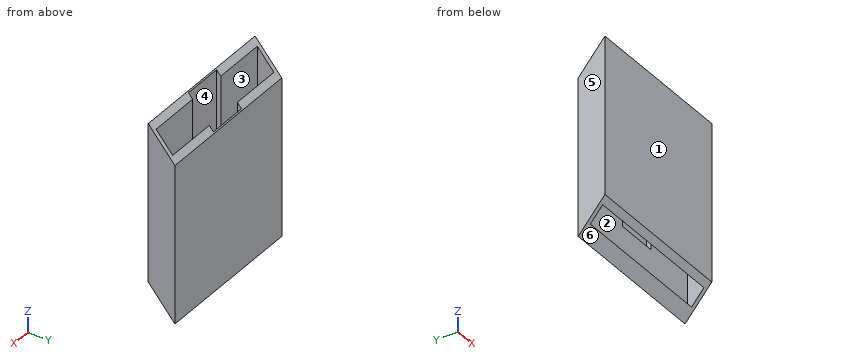
```python
from build123d import *

# Parameters (mm, degrees)
F1_DEPTH = 24.13
F2_W     = 12.7
F2_H     = 1.27
F3_DEPTH = 45.72
F4_DEPTH = 54.61


with BuildPart() as f1:
    # F0 (on Right) → F1 (new body, symmetric)
    with BuildSketch(Plane.YZ):
        Polygon((-16.67125, -9.728764), (-24.834652, 0), (-24.834652, -48.26), (-16.67125, -57.988764), align=None)
    extrude(amount=F1_DEPTH, both=True)

    # F2 (on Top) → F3 (cut)
    with BuildSketch(Plane.XY):
        with Locations((0, -17.577951)):
            Rectangle(F2_W, F2_H)
        with Locations((0, -23.927951)):
            Rectangle(F2_W, F2_H)
    extrude(amount=-F3_DEPTH, mode=Mode.SUBTRACT)

    # F2 (on Top) → F4 (cut)
    with BuildSketch(Plane.XY):
        Polygon((22.86, -23.292951), (22.86, -18.212951), (6.35, -18.212951), (-6.35, -18.212951), (-22.86, -18.212951), (-22.86, -23.292951), (-6.35, -23.292951), (6.35, -23.292951), align=None)
    extrude(amount=-F4_DEPTH, mode=Mode.SUBTRACT)


solid = f1.part
```
Here's how the part is built. I have some questions about the finished solid (model axes, mm). Face numbers are marked on the shaded views. A direction names the side the tool comes from. Round coordinates to 2 decimals unless told otherwise and drop trailing zeros. Order: outer loops, then holes, each group sorted by start corner. A loop starts at its lowest first (then second) coordinate and runs counter-clockwise, first axis right, second up. Notation, with made-up numbers: M 49,27.25 L 75,27.25 A25 ccw 75,45.25 Z; hole C 87,-23 d7. An arc over 180 degrees is marked long. One line per question, with ' | ' between items.
1) I want a section at B-B, the plane y = -21. Write out the boundary of the cut face in (x, z), then the cut area to 3 significant figures.
Working result:
outline: M -24.13,-52.83 L -22.86,-52.83 L -22.86,-4.57 L -24.13,-4.57 Z; M 22.86,-52.83 L 24.13,-52.83 L 24.13,-4.57 L 22.86,-4.57 Z | area: 123 mm²
2) For pin 1 Ø1 at (x, y) = (2, -24) entering from +Z, with a flat end and sliding along its axis, tell me the tip position at first contact or that it passes through.
Working result:
pin 1: z = -45.72
3) I want a section at D-D, the plane x = 1.5. Write out the boundary of the cut face in (y, z), then the cut area to 3 significant figures.
Working result:
outline: M -24.83,-48.26 L -23.29,-50.1 L -23.29,-45.72 L -24.56,-45.72 L -24.56,-0.32 L -24.83,0 Z; M -19.51,-54.61 L -16.67,-57.99 L -16.67,-9.73 L -16.94,-9.4 L -16.94,-45.72 L -18.21,-45.72 L -18.21,-54.61 Z | area: 46.0 mm²
4) I need wall thicknesses on line 1 along Y through (x, z) = (17.5, -34); line 2 along X through (y, z) = (-23.75, -43.5); line 3 along X through (y, z) = (-18.5, -40). Which ranges of each line are inside material? Lowest first, please.
Working result:
line 1: -24.83 to -23.29, -18.21 to -16.67 | line 2: -24.13 to -6.35, 6.35 to 24.13 | line 3: -24.13 to -22.86, 22.86 to 24.13
5) If we mould it in two halves opening along Y, with no side actions, what happens to the marked faces 4, 5 and 6? For each: +Y half, -Y half, draft (parallel to the pull), parting line (faces both ways), or undercut.
Working result:
face 4: undercut | face 5: draft | face 6: -Y half
6) For the marked faces 1, 2 and 3, which set-ups out of +Z, -Z, +X, -X, +Y, -Y let a thin tool reach every point of the face, with its end or its side?
Working result:
face 1: +Z, -Z, +X, -X, -Y | face 2: +Z | face 3: +Z, -Z
7) I want a section at A-A, the plane x = 12. Write out the boundary of the cut face in (y, z).
Working result:
outline: M -24.83,-48.26 L -23.29,-50.1 L -23.29,-1.84 L -24.83,0 Z; M -19.51,-54.61 L -16.67,-57.99 L -16.67,-9.73 L -18.21,-7.89 L -18.21,-54.61 Z
8) I want a section at C-C, the plane z = -31. Write out the boundary of the cut face in (x, y), then the cut area to 3 significant figures.
Working result:
outline: M -24.13,-24.83 L 24.13,-24.83 L 24.13,-16.67 L -24.13,-16.67 Z; hole M -22.86,-23.29 L -6.35,-23.29 L -6.35,-24.56 L 6.35,-24.56 L 6.35,-23.29 L 22.86,-23.29 L 22.86,-18.21 L 6.35,-18.21 L 6.35,-16.94 L -6.35,-16.94 L -6.35,-18.21 L -22.86,-18.21 Z | area: 129 mm²
